Here's how the part is built. I have some questions about the finished solid (model axes, mm). Face numbers are marked on the shaded views. Coordinates: 2 decimals unless noted, no trailing zeros. Write each loop counter-clockwise with the first axis right and the second up, starting at its lowest first coordinate (ties: lowest second). Pieces come first, ordered by that corner, then holes.
Item 1: I want a section at C-C (z = 3.5). Please give me the cut outline in (x, y).
Item 2: Please list where these lines run through material, in increasing order: line 1 (Y direction, x = 0, z = 4); line 2 (X direction, y = -137, z = 2.25); line 3 (Y direction, x = 1.5, z = 4.75).
Item 3: I want a section at A-A (y = 0). Please give me the cut outline in (x, z).
Item 4: I want a section at B-B (x = 0). Please give me the cut outline in (y, z).
Item 5: I want a section at D-D (y = -96). Please give me the cut outline in (x, z).
Item 6: If we mould it in two halves opening along X, with no side actions, what happens to the marked faces 1, 2 and 3? For each: pulls with the +X half, pulls with the -X half, needs draft (parallel to the pull), parting line crosses it, or undercut.
Item 7: I'm going to push flat-ended pins straight in: P1, Ø4, axis at y = -109.5, z = 4.5, coming from the +X side; P2, Ø4, axis at x = -13, z = 7, coming from the +Y side; P3, Ø3, axis at y = -21.5, z = 9, coming from the -X side; P4, Ø24, axis at x = 0, y = 0, coming from the +Z side. Where does each tip first touch, or does it pass through?
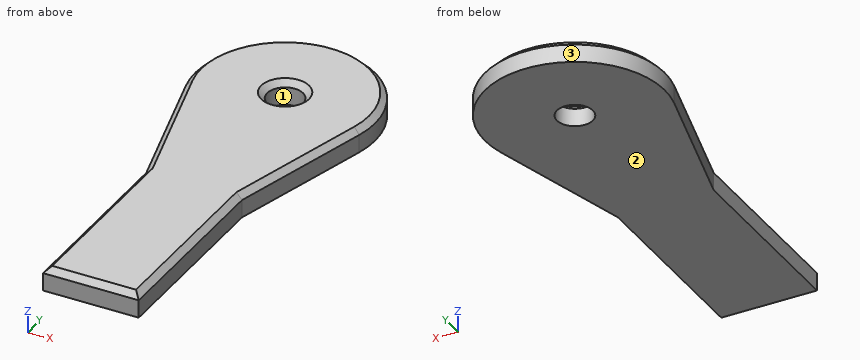
from build123d import *

# Parameters (mm, degrees)
SKETCH1_R           = 7.5
BOSS_EXTRUDE1_DEPTH = 10
CHAMFER1_SIZE       = 2.5


with BuildPart() as part:
    # Sketch1 → Boss-Extrude1 (new body)
    with BuildSketch(Plane.XY):
        with BuildLine():
            Line((36.222218486, -9.705714191), (20, -70.247857792))
            Line((20, -70.247857792), (20, -150))
            Line((20, -150), (-20, -150))
            Line((-20, -150), (-20, -70.247857792))
            Line((-20, -70.247857792), (-36.222218486, -9.705714191))
            ThreePointArc((-36.222218486, -9.705714191), (0, 37.5), (36.222218486, -9.705714191))
        make_face()
        Circle(SKETCH1_R, mode=Mode.SUBTRACT)
    extrude(amount=BOSS_EXTRUDE1_DEPTH)

    # Chamfer1
    chamfer1_edges = [part.edges().sort_by_distance(p)[0] for p in [
        (-20, -110.123928896, 10),
        (0, -150, 10),
        (-7.5, 0, 10),
        (20, -110.123928896, 10),
        (28.111109243, -39.976785992, 10),
        (0, 37.5, 10),
        (-28.111109243, -39.976785992, 10),
    ]]
    chamfer(chamfer1_edges, length=CHAMFER1_SIZE)


solid = part.part
Answer:
1. outline: (-36.22, -9.71) - (-20, -70.25) - (-20, -150) - (20, -150) - (20, -70.25) - (36.22, -9.71) arc R37.5 ccw (long way) to start; hole circle Ø15 at (0, 0)
2. line 1: y = -150 to -7.5, 7.5 to 37.5
2. line 2: x = -20 to 20
2. line 3: y = -150 to -7.35, 7.35 to 37.47
3. outline: (-37.5, 0) - (-7.5, 0) - (-7.5, 7.5) - (-10, 10) - (-35, 10) - (-37.5, 7.5) - close; (7.5, 0) - (37.5, 0) - (37.5, 7.5) - (35, 10) - (10, 10) - (7.5, 7.5) - close
4. outline: (-150, 0) - (-7.5, 0) - (-7.5, 7.5) - (-10, 10) - (-147.5, 10) - (-150, 7.5) - close; (7.5, 0) - (37.5, 0) - (37.5, 7.5) - (35, 10) - (10, 10) - (7.5, 7.5) - close
5. outline: (-20, 0) - (20, 0) - (20, 7.5) - (17.5, 10) - (-17.5, 10) - (-20, 7.5) - close
6. face 1: undercut
6. face 2: needs draft
6. face 3: parting line crosses it
7. P1: stops at x = 20
7. P2: stops at y = 35.85
7. P3: stops at x = -33.11
7. P4: stops at z = 10
